from build123d import *

# Parameters (mm, degrees)
EXTRUDE_1_DEPTH     = 4
SKETCH_2_R          = 3
EXTRUDE_2_DEPTH     = 16
CUT_EXTRUDE_1_DEPTH = 1.5
CUT_EXTRUDE_2_DEPTH = 4.5
CHAMFER_2_SIZE      = 1


with BuildPart() as part:
    # Эскиз1 → Бобышка-Вытянуть1 (new body, symmetric)
    with BuildSketch(Plane.XY):
        Polygon((8.25, 0), (-8.25, 0), (-8.25, 3.5), (-4, 3.5), (-4, 5), (4, 5), (4, 3.5), (8.25, 3.5), align=None)
    extrude(amount=EXTRUDE_1_DEPTH, both=True)

    # Эскиз2 → Бобышка-Вытянуть2 (add)
    with BuildSketch(Plane(origin=(0, 5, 0), x_dir=(1, 0, 0), z_dir=(0, 1, 0))):
        with Locations(Location((0, 0, 0), (0, 0, 270))):  # turned: the seam where the file's is
            Circle(SKETCH_2_R)
    extrude(amount=EXTRUDE_2_DEPTH)

    # Эскиз3 → Вырез-Вытянуть1 (cut)
    with BuildSketch(Plane(origin=(0, 5, 0), x_dir=(1, 0, 0), z_dir=(0, 1, 0))):
        with BuildLine():
            Line((-4, 0), (-4, 4))
            Line((-4, 4), (0, 4))
            ThreePointArc((0, 4), (-2.828427125, 2.828427125), (-4, 0))
        make_face()
        with BuildLine():
            Line((0, -4), (4, -4))
            Line((4, -4), (4, 0))
            ThreePointArc((4, 0), (2.828427125, -2.828427125), (0, -4))
        make_face()
    extrude(amount=-CUT_EXTRUDE_1_DEPTH, mode=Mode.SUBTRACT)

    # Эскиз4 → Вырез-Вытянуть2 (cut, through all)
    with BuildSketch(Plane(origin=(0, 3.5, 0), x_dir=(1, 0, 0), z_dir=(0, 1, 0))):
        with BuildLine():
            Line((-7.215434845, 4), (-8.25, 4))
            Line((-8.25, 4), (-8.25, 0))
            ThreePointArc((-8.25, 0), (-7.987172136, 2.065812495), (-7.215434845, 4))
        make_face()
        with BuildLine():
            Line((7.215434845, -4), (8.25, -4))
            Line((8.25, -4), (8.25, 0))
            ThreePointArc((8.25, 0), (7.987172136, -2.065812495), (7.215434845, -4))
        make_face()
    extrude(amount=-CUT_EXTRUDE_2_DEPTH, mode=Mode.SUBTRACT)

    # Вырез-По траектории1: sweep along a path in Эскиз6
    with BuildLine(Plane.XZ) as sweep_1_path:
        Line((0, -8.25), (8.25, -8.25))
        Line((8.25, -8.25), (8.25, 0))
        ThreePointArc((8.25, 0), (5.833630945, 5.833630945), (0, 8.25))
        Line((0, 8.25), (-8.25, 8.25))
        Line((-8.25, 8.25), (-8.25, 0))
        ThreePointArc((-8.25, 0), (-5.833630945, -5.833630945), (0, -8.25))
    # Эскиз5 → Вырез-По траектории1 (sweep, cut)
    with BuildSketch(Plane.XY.offset(4)):
        Polygon((-8.25, 2), (-4.8, 0), (-8.25, 0), align=None)
    sweep(path=sweep_1_path.line, transition=Transition.RIGHT, mode=Mode.SUBTRACT)

    # Фаска2
    chamfer_2_edges = [part.edges().sort_by_distance(p)[0] for p in [
        (0, 21, -3),
    ]]
    chamfer(chamfer_2_edges, length=CHAMFER_2_SIZE)


solid = part.part
Could you check a few things on this model? Use its own coordinates, in mm. A direction names the side the tool comes from. Round coordinates to 2 decimals unless told otherwise and drop trailing zeros. Order: outer loops, then holes, each group sorted by start corner. A loop starts at its lowest first (then second) coordinate and runs counter-clockwise, first axis right, second up.
(1) Which directions (+Z, -Z, +X, -X, +Y, -Y) give clear straight access to the entire face, cutting with the end or side of a thin tool? Please do faces 1 (the cylindrical face through (2.859, 4.26, 2.797)), 2 (the flat face through (-4, 4, 2)), 3 (the flat face through (2, 5, -3)), 4 (the cylindrical face through (-2.797, 4.26, -2.859)).
Response values:
face 1: +Z, +X, +Y
face 2: +Z, -Z, -X, +Y
face 3: +Y
face 4: -Z, -X, +Y
(2) Please list where these lines run through material, in increasing order: line 1 along Y through (x, z) = (3, -1.25); line 2 along X through (y, z) = (3.25, -0.25); line 3 along Y through (x, z) = (3, 3.25).
Response values:
line 1: y = 0 to 5
line 2: x = -8.25 to 8.25
line 3: y = 0 to 3.5
(3) I'm going to push flat-ended pins straight in: pin 1 (2.5 mm diameter, centred on x = -2.5, z = -1, fed in from +Y); pin 2 (4 mm diameter, centred on x = -1.5, y = 17.5, fed in from -Z). Where does each tip first touch, or does it pass through?
Response values:
pin 1: stops at y = 21
pin 2: stops at z = -3
(4) Imagine slicing it at A-A (y = 4.5). Write out the boundary of the cut face in (x, z).
Response values:
outline: (-4, 0) arc R4 ccw to (0, -4) - (4, -4) - (4, 0) arc R4 ccw to (0, 4) - (-4, 4) - close
(5) Imagine slicing it at B-B (y = 10.5). Write out the boundary of the cut face in (x, z).
Response values:
outline: circle Ø6 at (0, 0)
